The drawing under review shows one solid part. Ordinate dimensions are in mm from its lowest x, y, z. Coordinates: 2 decimals unless noted, no trailing zeros. Order: outer loops, then holes, each group sorted by start corner. A loop starts at its lowest first (then second) coordinate and runs counter-clockwise, first axis right, second up. Notation, with made-up numbers: M 20.25,58 L 57.25,58 A37 cw 57.25,94 Z; hole C 66.25,58 d4. An arc over 180 degrees is marked long. Answer as a JSON object with one key per item and string values.
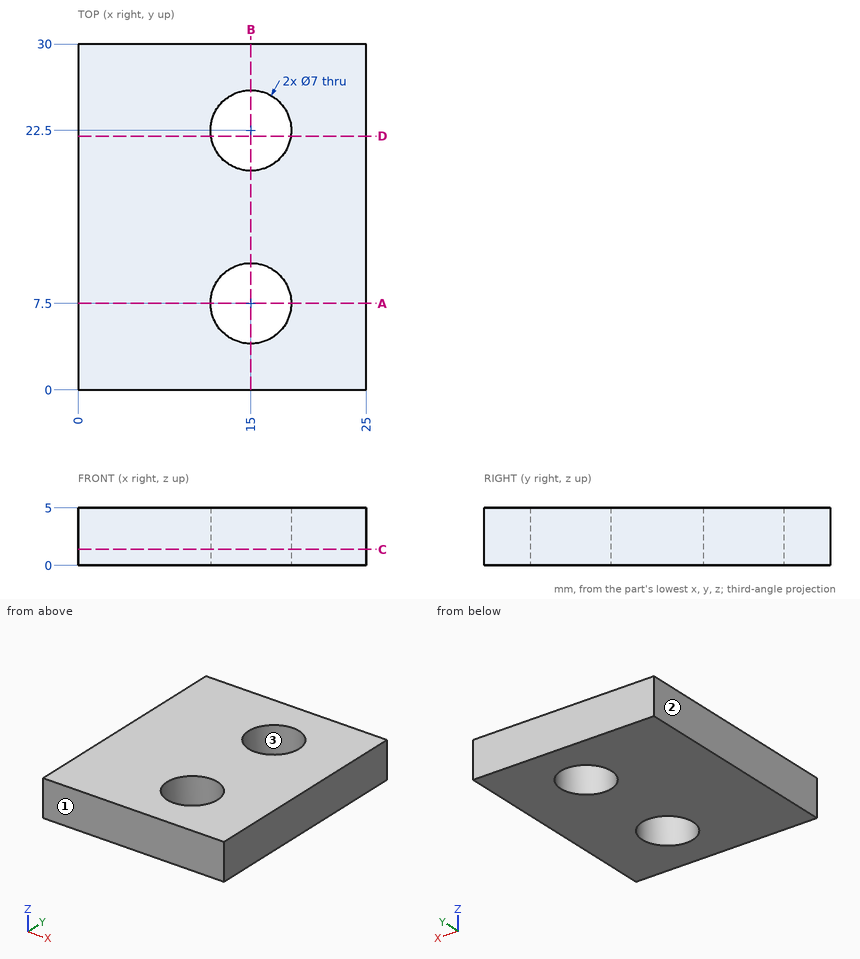
1) Add section B-B (x = 15). State the section outline as (y, z) points.
Taken from the geometry:
{"outline": "M 0,0 L 4,0 L 4,5 L 0,5 Z; M 11,0 L 19,0 L 19,5 L 11,5 Z; M 26,0 L 30,0 L 30,5 L 26,5 Z"}
2) To check wall thickness, follow L1, parallel to Y at x = 15, z = 1; L2, parallel to X at y = 22.5, z = 2; L3, parallel to X at y = 20, z = 1.9. State the ranges of each line that lie inside material, in increasing order.
Taken from the geometry:
{"L1": "y = 0 to 4, 11 to 19, 26 to 30", "L2": "x = 0 to 11.5, 18.5 to 25", "L3": "x = 0 to 12.55, 17.45 to 25"}
3) Add section C-C (z = 1.4). State the section outline as (x, y) points, and give its area (3 significant figures).
Taken from the geometry:
{"outline": "M 0,0 L 25,0 L 25,30 L 0,30 Z; hole C 15,7.5 d7; hole C 15,22.5 d7", "area": "673 mm2"}
4) Mouldability with a two-part tool opening along X and no side actions: class the marked faces 1, 2 and 3 as released by +X, released by -X, zero draft, split by the parting line, or undercut.
Taken from the geometry:
{"face 1": "zero draft", "face 2": "released by -X", "face 3": "undercut"}
5) Add section D-D (y = 22). State the section outline as (x, z) points, and give its area (3 significant figures).
Taken from the geometry:
{"outline": "M 0,0 L 11.54,0 L 11.54,5 L 0,5 Z; M 18.46,0 L 25,0 L 25,5 L 18.46,5 Z", "area": "90.4 mm2"}
6) Add section A-A (y = 7.5). State the section outline as (x, z) points.
Taken from the geometry:
{"outline": "M 0,0 L 11.5,0 L 11.5,5 L 0,5 Z; M 18.5,0 L 25,0 L 25,5 L 18.5,5 Z"}
